CAD build for the part. Positions are in the model's coordinates, mm. Face numbers are marked on the shaded views. A direction names the side the tool comes from. Coordinates: 2 decimals unless noted, no trailing zeros. Order: outer loops, then holes, each group sorted by start corner. A loop starts at its lowest first (then second) coordinate and runs counter-clockwise, first axis right, second up. Notation, with made-up numbers: (48, -40) - (89, -40) arc R3 ccw to (89, -36) - close; hole circle Ø3 at (81.25, -26.75). An arc over 180 degrees is marked (long way). Return JSON: item names as keys, results as strings.
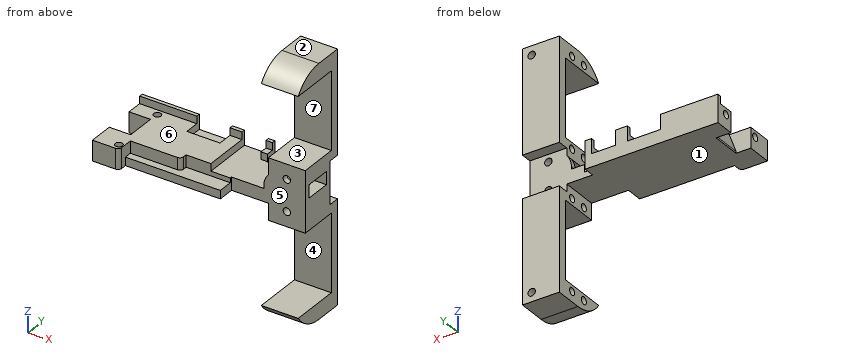
from build123d import *

# Parameters (mm, degrees)
BOSS_EXTRUDE1_DEPTH = 35
CUT_EXTRUDE1_REACH  = 164.604
SKETCH2_W           = 42
SKETCH2_H           = 21
SKETCH3_R           = 2
CUT_EXTRUDE2_DEPTH  = 10
FILLET1_R           = 20
CUT_EXTRUDE5_REACH  = 164.604
SKETCH6_W           = 42
SKETCH6_H           = 9
SKETCH7_R           = 2
CUT_EXTRUDE6_DEPTH  = 12
CUT_EXTRUDE7_DEPTH  = 9
SKETCH9_R           = 2
CUT_EXTRUDE8_DEPTH  = 10
CUT_EXTRUDE9_DEPTH  = 6
SKETCH11_R          = 2
CUT_EXTRUDE10_DEPTH = 9
SKETCH12_R          = 2
CUT_EXTRUDE11_DEPTH = 10
SKETCH14_W          = 83
SKETCH14_H          = 33
CUT_EXTRUDE13_DEPTH = 4
CUT_EXTRUDE14_DEPTH = 6.5
SKETCH16_W          = 14.5
SKETCH16_H          = 11
BOSS_EXTRUDE2_DEPTH = 5
SKETCH13_R          = 2
CUT_EXTRUDE12_DEPTH = 12
FILLET2_R           = 2
FILLET3_R           = 2
SKETCH17_W          = 18
SKETCH17_H          = 10
CUT_EXTRUDE15_DEPTH = 8
CUT_EXTRUDE18_REACH = 104.86
SKETCH20_W          = 8
SKETCH20_H          = 16
CHAMFER1_SIZE       = 10
CHAMFER1_SIZE2      = 3.639702343
CUT_EXTRUDE19_REACH = 164.604
SKETCH22_W          = 7
SKETCH22_H          = 14
FILLET8_R           = 10


with BuildPart() as part:
    # Sketch1 → Boss-Extrude1 (new body)
    with BuildSketch(Plane(origin=(0, 0, 0), x_dir=(1, 0, 0), z_dir=(0, 1, 0))):
        Polygon((-40.317617866, 43.23325062), (45.682382134, 43.23325062), (45.682382134, -16.76674938), (65.682382134, -16.76674938), (65.682382134, 118.23325062), (45.682382134, 118.23325062), (45.682382134, 58.23325062), (-40.317617866, 58.23325062), align=None)
    extrude(amount=BOSS_EXTRUDE1_DEPTH)

    # Sketch2 → Cut-Extrude1 (cut, up to next)
    with BuildSketch(Plane(origin=(65.682382134, 0, 0), x_dir=(0, 0, -1), z_dir=(1, 0, 0)), mode=Mode.PRIVATE) as cut_extrude1_sk1:
        with Locations((13.23325062, 19.5)):
            Rectangle(SKETCH2_W, SKETCH2_H)
    cut_extrude1_tool1 = extrude(cut_extrude1_sk1.sketch, amount=-CUT_EXTRUDE1_REACH, mode=Mode.PRIVATE) & part.part
    # Sketch2 → Cut-Extrude1 (cut, up to next)
    with BuildSketch(Plane(origin=(65.682382134, 0, 0), x_dir=(0, 0, -1), z_dir=(1, 0, 0)), mode=Mode.PRIVATE) as cut_extrude1_sk2:
        with Locations((88.23325062, 19.5)):
            Rectangle(SKETCH2_W, SKETCH2_H)
    cut_extrude1_tool2 = extrude(cut_extrude1_sk2.sketch, amount=-CUT_EXTRUDE1_REACH, mode=Mode.PRIVATE) & part.part
    add(cut_extrude1_tool1.solids().sort_by_distance((65.682382, 19.5, -13.233251))[0], mode=Mode.SUBTRACT)
    add(cut_extrude1_tool2.solids().sort_by_distance((65.682382, 19.5, -88.233251))[0], mode=Mode.SUBTRACT)

    # Sketch3 → Cut-Extrude2 (cut)
    with BuildSketch(Plane.ZY.offset(-45.682382134)):
        with Locations((11.26674938, 24.75)):
            Circle(SKETCH3_R)
        with Locations((11.26674938, 15.25)):
            Circle(SKETCH3_R)
        with Locations((-37.73325062, 24.75)):
            Circle(SKETCH3_R)
        with Locations((-37.73325062, 15.25)):
            Circle(SKETCH3_R)
        with Locations(Location((-112.73325062, 24.75, 0), (0, 0, 180))):
            Circle(SKETCH3_R)
        with Locations(Location((-112.73325062, 15.25, 0), (0, 0, 180))):
            Circle(SKETCH3_R)
        with Locations(Location((-63.73325062, 15.25, 0), (0, 0, 180))):
            Circle(SKETCH3_R)
        with Locations(Location((-63.73325062, 24.75, 0), (0, 0, 180))):
            Circle(SKETCH3_R)
    extrude(amount=-CUT_EXTRUDE2_DEPTH, mode=Mode.SUBTRACT)

    # Fillet1
    fillet1_edges = [part.edges().sort_by_distance(p)[0] for p in [
        (55.682382134, 0, -118.23325062),
        (55.682382134, 0, 16.76674938),
    ]]
    fillet(fillet1_edges, radius=FILLET1_R)

    # Sketch6 → Cut-Extrude5 (cut, up to next)
    with BuildSketch(Plane(origin=(65.682382134, 0, 0), x_dir=(0, 0, -1), z_dir=(1, 0, 0)), mode=Mode.PRIVATE) as cut_extrude5_sk1:
        with Locations((13.23325062, 4.5)):
            Rectangle(SKETCH6_W, SKETCH6_H)
    cut_extrude5_tool1 = extrude(cut_extrude5_sk1.sketch, amount=-CUT_EXTRUDE5_REACH, mode=Mode.PRIVATE) & part.part
    # Sketch6 → Cut-Extrude5 (cut, up to next)
    with BuildSketch(Plane(origin=(65.682382134, 0, 0), x_dir=(0, 0, -1), z_dir=(1, 0, 0)), mode=Mode.PRIVATE) as cut_extrude5_sk2:
        with Locations((88.23325062, 4.5)):
            Rectangle(SKETCH6_W, SKETCH6_H)
    cut_extrude5_tool2 = extrude(cut_extrude5_sk2.sketch, amount=-CUT_EXTRUDE5_REACH, mode=Mode.PRIVATE) & part.part
    add(cut_extrude5_tool1.solids().sort_by_distance((65.682382, 4.5, -13.233251))[0], mode=Mode.SUBTRACT)
    add(cut_extrude5_tool2.solids().sort_by_distance((65.682382, 4.5, -88.233251))[0], mode=Mode.SUBTRACT)

    # Sketch7 → Cut-Extrude6 (cut)
    with BuildSketch(Plane.ZY.offset(40.317617866)):
        with Locations((-50.73325062, 28.5)):
            Circle(SKETCH7_R)
        with Locations((-50.73325062, 5)):
            Circle(SKETCH7_R)
    extrude(amount=-CUT_EXTRUDE6_DEPTH, mode=Mode.SUBTRACT)

    # Sketch8 → Cut-Extrude7 (cut)
    with BuildSketch(Plane.XZ):
        Polygon((45.682382134, -67.23325062), (45.682382134, -58.23325062), (25.682382134, -58.23325062), (25.682382134, -43.23325062), (45.682382134, -43.23325062), (45.682382134, -34.23325062), (65.682382134, -34.23325062), (65.682382134, -67.23325062), align=None)
    extrude(amount=-CUT_EXTRUDE7_DEPTH, mode=Mode.SUBTRACT)

    # Sketch9 → Cut-Extrude8 (cut)
    with BuildSketch(Plane.XZ.offset(-9)):
        with Locations(Location((55.682382134, -42.23325062, 0), (0, 0, 270))):
            Circle(SKETCH9_R)
        with Locations(Location((55.682382134, -59.23325062, 0), (0, 0, 270))):
            Circle(SKETCH9_R)
    extrude(amount=-CUT_EXTRUDE8_DEPTH, mode=Mode.SUBTRACT)

    # Sketch10 → Cut-Extrude9 (cut)
    with BuildSketch(Plane(origin=(0, 35, 0), x_dir=(1, 0, 0), z_dir=(0, 1, 0))):
        Polygon((45.682382134, 62.23325062), (65.682382134, 62.23325062), (65.682382134, 39.23325062), (45.682382134, 39.23325062), (45.682382134, 43.23325062), (31.682382134, 43.23325062), (31.682382134, 58.23325062), (45.682382134, 58.23325062), align=None)
    extrude(amount=-CUT_EXTRUDE9_DEPTH, mode=Mode.SUBTRACT)

    # Sketch11 → Cut-Extrude10 (cut)
    with BuildSketch(Plane(origin=(0, 29, 0), x_dir=(1, 0, 0), z_dir=(0, 1, 0))):
        with Locations(Location((55.682382134, 58.23325062, 0), (0, 0, 270))):
            Circle(SKETCH11_R)
        with Locations(Location((55.682382134, 43.23325062, 0), (0, 0, 270))):
            Circle(SKETCH11_R)
    extrude(amount=-CUT_EXTRUDE10_DEPTH, mode=Mode.SUBTRACT)

    # Sketch12 → Cut-Extrude11 (cut)
    with BuildSketch(Plane(origin=(0, 35, 0), x_dir=(1, 0, 0), z_dir=(0, 1, 0))):
        with Locations(Location((60.682382134, -11.76674938, 0), (0, 0, 270))):
            Circle(SKETCH12_R)
        with Locations(Location((60.682382134, 113.23325062, 0), (0, 0, 270))):
            Circle(SKETCH12_R)
    extrude(amount=-CUT_EXTRUDE11_DEPTH, mode=Mode.SUBTRACT)

    # Sketch14 → Cut-Extrude13 (cut)
    with BuildSketch(Plane.XY.offset(-43.23325062)):
        with Locations((1.182382134, 16.5)):
            Rectangle(SKETCH14_W, SKETCH14_H)
    extrude(amount=-CUT_EXTRUDE13_DEPTH, mode=Mode.SUBTRACT)

    # Sketch15 → Cut-Extrude14 (cut)
    with BuildSketch(Plane.XY.offset(-47.23325062)):
        Polygon((1.682382134, 8), (33.682382134, 8), (33.682382134, 0), (-25.817617866, 0), (-25.817617866, 4), (1.682382134, 4), align=None)
    extrude(amount=-CUT_EXTRUDE14_DEPTH, mode=Mode.SUBTRACT)

    # Sketch16 → Boss-Extrude2 (add)
    with BuildSketch(Plane.XZ):
        with Locations((-33.067617866, -52.73325062)):
            Rectangle(SKETCH16_W, SKETCH16_H)
    extrude(amount=BOSS_EXTRUDE2_DEPTH)

    # Sketch13 → Cut-Extrude12 (cut)
    with BuildSketch(Plane.XY.offset(-43.23325062)):
        with Locations((-28.317617866, 29.5)):
            Circle(SKETCH13_R)
        with Locations((34.182382134, 29.5)):
            Circle(SKETCH13_R)
        with Locations((34.182382134, -1.5)):
            Circle(SKETCH13_R)
        with Locations((-28.317617866, -1.5)):
            Circle(SKETCH13_R)
    extrude(amount=-CUT_EXTRUDE12_DEPTH, mode=Mode.SUBTRACT)

    # Fillet2
    fillet2_edges = [part.edges().sort_by_distance(p)[0] for p in [
        (-25.817617866, -5, -52.73325062),
    ]]
    fillet(fillet2_edges, radius=FILLET2_R)

    # Fillet3
    fillet3_edges = [part.edges().sort_by_distance(p)[0] for p in [
        (1.682382134, 4, -50.48325062),
    ]]
    fillet(fillet3_edges, radius=FILLET3_R)

    # Sketch17 → Cut-Extrude15 (cut)
    with BuildSketch(Plane.XY.offset(-43.23325062)):
        Polygon((43.182382134, -5), (15.182382134, -5), (15.182382134, 35), (28.182382134, 35), (28.182382134, 29), (43.182382134, 29), align=None)
        with Locations((-0.317617866, 30)):
            Rectangle(SKETCH17_W, SKETCH17_H)
    extrude(amount=-CUT_EXTRUDE15_DEPTH, mode=Mode.SUBTRACT)

    # Sketch20 → Cut-Extrude18 (cut, up to next)
    with BuildSketch(Plane.XY.offset(-47.23325062), mode=Mode.PRIVATE) as cut_extrude18_sk1:
        with Locations((-36.317617866, 16.5)):
            Rectangle(SKETCH20_W, SKETCH20_H)
    cut_extrude18_tool1 = extrude(cut_extrude18_sk1.sketch, amount=-CUT_EXTRUDE18_REACH, mode=Mode.PRIVATE) & part.part
    add(cut_extrude18_tool1.solids().sort_by_distance((-36.317618, 16.5, -47.233251))[0], mode=Mode.SUBTRACT)

    # Chamfer1
    chamfer1_edges = [part.edges().sort_by_distance(p)[0] for p in [
        (-32.317617866, 16.5, -47.23325062),
    ]]
    chamfer1_side = [part.faces().sort_by_distance(p)[0] for p in [
        (-32.317617866, 16.5, -52.73325062),
    ]]
    chamfer(chamfer1_edges, length=CHAMFER1_SIZE, length2=CHAMFER1_SIZE2, reference=chamfer1_side[0])

    # Sketch22 → Cut-Extrude19 (cut, up to next)
    with BuildSketch(Plane(origin=(65.682382134, 0, 0), x_dir=(0, 0, -1), z_dir=(1, 0, 0)), mode=Mode.PRIVATE) as cut_extrude19_sk1:
        with Locations((46.73325062, 19)):
            Rectangle(SKETCH22_W, SKETCH22_H)
    cut_extrude19_tool1 = extrude(cut_extrude19_sk1.sketch, amount=-CUT_EXTRUDE19_REACH, mode=Mode.PRIVATE) & part.part
    add(cut_extrude19_tool1.solids().sort_by_distance((65.682382, 19, -46.733251))[0], mode=Mode.SUBTRACT)

    # Fillet8
    # the kernel refuses this fillet: 10 mm, written as the material it takes off along each edge
    with BuildSketch(Plane(origin=(43.182382134, 28.535945694, -43.23325062), x_dir=(0, 0, -1), z_dir=(0, -1, 0)), Plane(origin=(43.182382134, 45.535945694, -43.23325062), x_dir=(0, 0, -1), z_dir=(0, -1, 0))) as fillet8_piece_1:
        with BuildLine():
            CenterArc((6.614378278, 10), FILLET8_R, 228.590377891, 41.409622109)
            Line((0, 2.5), (0, 0))
            Line((0, 0), (6.614378278, 0))
        make_face()
    extrude(amount=36.071891388, mode=Mode.SUBTRACT)


solid = part.part
Item 1: Band-saw the part on D-D, the plane y = 15.25. Count the separate pieces of the cut face and the enclosed holes in it, then the cut area to 3 significant figures.
Findings below:
{"separate pieces": "4", "enclosed holes": "1", "area": "1,390 mm²"}
Item 2: Mould opens along Z. For the marked faces 1, 2, 3 and 4 say: released by +Z, released by -Z, zero draft, split by the parting line, or undercut.
Findings below:
{"face 1": "released by -Z", "face 2": "released by +Z", "face 3": "undercut", "face 4": "undercut"}
Item 3: Band-saw the part on A-A, the plane x = -21.5. List the corners of the cut face in (y, z).
Findings below:
{"outline": "(0, -58.23) - (35, -58.23) - (35, -43.23) - (33, -43.23) - (33, -47.23) - (4, -47.23) - (4, -53.73) - (0, -53.73) - close"}
Item 4: Which spindle directions (+Z, -Z, +X, -X, +Y, -Y) get a long thin tool onto all of the face, cutting with end or side? Do the marked faces 5, 6 and 7. Say none if no direction does.
Findings below:
{"face 5": "+X, -Y", "face 6": "+Z, -X, -Y", "face 7": "+X, -X, -Y"}
Item 5: Band-saw the part on C-C, the plane z = -12. List the corners of the cut face in (x, y).
Findings below:
{"outline": "(45.68, 30) - (65.68, 30) - (65.68, 35) - (45.68, 35) - close"}
Item 6: Band-saw the part on B-B, the plane y = -1.5. List the corners of the cut face in (x, z), then the cut area to 4 significant figures.
Findings below:
{"outline": "(-40.32, -58.23) - (-25.82, -58.23) - (-25.82, -47.23) - (-26.32, -47.23) - (-26.32, -55.23) - (-30.32, -55.23) - (-30.32, -47.23) - (-40.32, -47.23) - close", "area": "127.5 mm²"}
Item 7: Wall check: L1, parallel to Z at x = -34.5, y = 4; L2, parallel to Z at x = 25, y = 16; L3, parallel to Z at x = -17.5, y = 13. Give the ranges that are in metal, low to high. Write a range as [from, to].
Findings below:
{"L1": "z = [-58.23, -52.47], [-49, -47.23]", "L2": "z = [-58.23, -51.23]", "L3": "z = [-58.23, -47.23]"}
Item 8: Drop flat-ended pins along their axis: P1, Ø1.2, axis at x = -20.5, z = -44.5, coming from the -Y side; P2, Ø1.5, axis at x = -8, y = 17, coming from the +Z side; P3, Ø12, axis at y = 10.5, z = 2.5, coming from the -X side. Give the stop position or say it passes through.
Findings below:
{"P1": "stops at y = 33", "P2": "stops at z = -47.23", "P3": "stops at x = 45.68"}
